```python
from build123d import *

# Parameters (mm, degrees)
F0_W        = 100
F0_H        = 50
F1_DEPTH    = 25
F2_R        = 15
F3_DEPTH    = 25.001
F4_T1_DEPTH = 75
F4_T3_DEPTH = 125


# Not quite as in the source:
# - a fillet or chamfer that OpenCascade refuses, or shapes differently, is made with other operations: its cross-section is extruded or revolved along the edge and cut away or added


with BuildPart() as f1:
    # F0 (on Top) → F1 (new body)
    with BuildSketch(Plane.XY):
        with Locations((50, 25)):
            Rectangle(F0_W, F0_H)
    extrude(amount=F1_DEPTH)

    # F2 (on face) → F3 (cut, through all)
    with BuildSketch(Plane.XY.offset(25)):
        with Locations((20, 20)):
            Circle(F2_R)
    extrude(amount=-F3_DEPTH, mode=Mode.SUBTRACT)

    # F4: fillet of radius 5 on 5 edges, made by hand

    # F4_s2 → F4_t1 (cut)
    with BuildSketch(Plane.XZ.offset(-62.5)):
        with BuildLine():
            ThreePointArc((0, 20), (1.4644660941, 23.5355339059), (5, 25))
            Line((5, 25), (0, 25))
            Line((0, 25), (0, 20))
        make_face()
        with BuildLine():
            ThreePointArc((95, 25), (98.5355339059, 23.5355339059), (100, 20))
            Line((100, 20), (100, 25))
            Line((100, 25), (95, 25))
        make_face()
    extrude(amount=F4_T1_DEPTH, mode=Mode.SUBTRACT)

    # F4_s4 → F4_t3 (cut)
    with BuildSketch(Plane.YZ.offset(-12.5)):
        with BuildLine():
            ThreePointArc((50, 20), (48.5355339059, 23.5355339059), (45, 25))
            Line((45, 25), (50, 25))
            Line((50, 25), (50, 20))
        make_face()
        with BuildLine():
            ThreePointArc((0, 20), (1.4644660941, 23.5355339059), (5, 25))
            Line((5, 25), (0, 25))
            Line((0, 25), (0, 20))
        make_face()
    extrude(amount=F4_T3_DEPTH, mode=Mode.SUBTRACT)

    # F4_s5 → F4_t6 (revolve, cut)
    with BuildSketch(Plane.XZ.offset(-20)):
        with BuildLine():
            ThreePointArc((40, 25), (36.4644660941, 23.5355339059), (35, 20))
            Line((35, 20), (35, 25))
            Line((35, 25), (40, 25))
        make_face()
    revolve(axis=Axis((20, 20, 25), (0, 0, 1)), mode=Mode.SUBTRACT)


solid = f1.part
```
CAD build for the part. Positions are in the model's coordinates, mm. Give positions to 0.01 mm unless a question says otherwise; leave off trailing zeros. Order: outer loops, then holes, each group sorted by start corner. A loop starts at its lowest first (then second) coordinate and runs counter-clockwise, first axis right, second up.
(1) Saw through at B-B, the plane z = 2.5. Give the cut face in (x, y), then the cut area to 3 significant figures.
(2) Flat gauge pin, fed straight in: pin 1 (10 mm diameter, centred on x = 19.5, y = 32.5, fed in from +Z). Where does the tip first touch, or does it go through?
(3) Saw through at A-A, the plane y = 20. Give the cut face in (x, z), then the cut area to 3 significant figures.
(4) Saw through at D-D, the plane z = 23.5. Give the cut face in (x, y).
(5) Drill centre lines: L1, parallel to Y at x = 20, z = 6; L2, parallel to Y at x = 15, z = 23; L3, parallel to X at y = 19, z = 8. Where is each one in solid material? Low to high.
(6) Mould opens along X. For faces 1 (the cylindrical face through (16.748, 5.357, 10.14)), 2 (the flat face through (5.5, 5.5, 25)), 3 (the cylindrical face through (1, 25, 23)) say: released by +X, released by -X, zero draft, split by the parting line, or undercut.
(7) Saw through at C-C, the plane x = 20. Give the cut face in (y, z).
Results found:
1. outline: (0, 0) - (100, 0) - (100, 50) - (0, 50) - close; hole circle Ø30 at (20, 20)
1. area: 4,290 mm2
2. pin 1: stops at z = 24.34
3. outline: (0, 0) - (5, 0) - (5, 20) arc R5 ccw to (2.5, 24.33) arc R5 ccw to (0, 20) - close; (35, 0) - (100, 0) - (100, 20) arc R5 ccw to (95, 25) - (40, 25) arc R5 ccw to (35, 20) - close
3. area: 1,730 mm2
4. outline: (1.43, 1.43) - (98.57, 1.43) - (98.57, 48.57) - (1.43, 48.57) - close; hole circle Ø32.86 at (20, 20)
5. L1: y = 0 to 5, 35 to 50
5. L2: y = 1 to 4.8, 35.2 to 49
5. L3: x = 0 to 5.03, 34.97 to 100
6. face 1: undercut
6. face 2: zero draft
6. face 3: released by -X
7. outline: (0, 0) - (5, 0) - (5, 20) arc R5 ccw to (2.5, 24.33) arc R5 ccw to (0, 20) - close; (35, 0) - (50, 0) - (50, 20) arc R5 ccw to (45, 25) - (40, 25) arc R5 ccw to (35, 20) - close
